```python
from build123d import *

# Parameters (mm, degrees)
F0_R     = 4.7879
F1_DEPTH = 15
F4_D     = 4.1
F5_D     = 4.1


with BuildPart() as f1:
    # F0 (on Top) → F1 (new body)
    with BuildSketch(Plane.XY):
        with BuildLine():
            ThreePointArc((-9.7879, 0), (0, 9.7879), (9.7879, 0))
            Line((9.7879, 0), (9.7879, 17.5))
            Line((9.7879, 17.5), (21.7879, 17.5))
            Line((21.7879, 17.5), (21.7879, 20))
            Line((21.7879, 20), (0, 20))
            Line((0, 20), (-21.7879, 20))
            Line((-21.7879, 20), (-21.7879, 17.5))
            Line((-21.7879, 17.5), (-9.7879, 17.5))
            Line((-9.7879, 17.5), (-9.7879, 0))
        make_face()
        with BuildLine():
            ThreePointArc((-9.7879, 0), (0, -9.7879), (9.7879, 0))
            ThreePointArc((9.7879, 0), (0, 9.7879), (-9.7879, 0))
        make_face()
        Circle(F0_R, mode=Mode.SUBTRACT)
    extrude(amount=F1_DEPTH)

    # F4 (through all)
    with Locations(Plane.XZ.offset(-17.5)):
        with Locations((15.7879, 7.5)):
            Hole(F4_D / 2)

    # F5 (through all)
    with Locations(Plane.XZ.offset(-17.5)):
        with Locations((-15.7879, 7.5)):
            Hole(F5_D / 2)


solid = f1.part
```
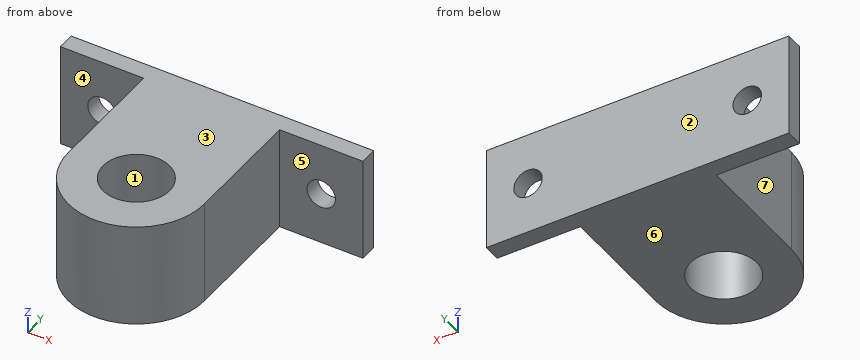
Design review of the part built by this model. Coordinates are the model's own, in mm. Face numbers are marked on the shaded views. A direction names the side the tool comes from. Coordinates: 2 decimals unless noted, no trailing zeros. Write each loop counter-clockwise with the first axis right and the second up, starting at its lowest first coordinate (ties: lowest second). Pieces come first, ordered by that corner, then holes.
1) Add section D-D (y = 2.5). Write out the cut boundary in (x, z).
2) Add section B-B (x = 0). Write out the cut boundary in (y, z).
3) Machinability: for the marked faces 5, 6 and 7, which of the approach directions +Z, -Z, +X, -X, +Y, -Y give a long, thin tool a straight path to every point of the face, cutting with its end or side? Answer none if there is none.
4) Add section C-C (z = 3). Write out the cut boundary in (x, y), plus the area to 3 significant figures.
5) To check wall thickness, follow L1, parallel to Y at x = 0, z = 4.25; L2, parallel to X at y = 2, z = 10.25; L3, parallel to Y at x = 19.5, z = 13. State the ranges of each line that lie inside material, in increasing order.
6) Mouldability with a two-part tool opening along Y and no side actions: class the marked faces 1, 2, 3 and 4 as +Y half, -Y half, draft (parallel to the pull), parting line (faces both ways), or undercut.
7) Add section A-A (z = 7.5). Write out the cut boundary in (x, y).
8) Insertion check: pin 1 (5 mm diameter, centred on x = 7, z = 8.5, fed in from -Y); pin 2 (4 mm diameter, centred on y = 17, z = 5.5, fed in from -X); pin 3 (6 mm diameter, centred on x = -17.5, z = 10.5, fed in from -Y); pin 4 (4 mm diameter, centred on y = 1.5, z = 2.5, fed in from -X). Each pin has a flat end and moves straight along its axis. Give the tip position at first contact, or say it passes through.
Check result:
1. outline: (-9.79, 0) - (-4.08, 0) - (-4.08, 15) - (-9.79, 15) - close; (4.08, 0) - (9.79, 0) - (9.79, 15) - (4.08, 15) - close
2. outline: (-9.79, 0) - (-4.79, 0) - (-4.79, 15) - (-9.79, 15) - close; (4.79, 0) - (20, 0) - (20, 15) - (4.79, 15) - close
3. face 5: +Z, -Z, +X, -Y
3. face 6: -Z, +X, -X, +Y, -Y
3. face 7: +Z, -Z, -X, -Y
4. outline: (-21.79, 17.5) - (-9.79, 17.5) - (-9.79, 0) arc R9.79 ccw to (9.79, 0) - (9.79, 17.5) - (21.79, 17.5) - (21.79, 20) - (-21.79, 20) - close; hole circle Ø9.58 at (0, 0)
4. area: 530 mm2
5. L1: y = -9.79 to -4.79, 4.79 to 20
5. L2: x = -9.79 to -4.35, 4.35 to 9.79
5. L3: y = 17.5 to 20
6. face 1: undercut
6. face 2: +Y half
6. face 3: draft
6. face 4: -Y half
7. outline: (-21.79, 17.5) - (-17.84, 17.5) - (-17.84, 20) - (-21.79, 20) - close; (-13.74, 17.5) - (-9.79, 17.5) - (-9.79, 0) arc R9.79 ccw to (9.79, 0) - (9.79, 17.5) - (13.74, 17.5) - (13.74, 20) - (-13.74, 20) - close; (17.84, 17.5) - (21.79, 17.5) - (21.79, 20) - (17.84, 20) - close; hole circle Ø9.58 at (0, 0)
8. pin 1: stops at y = -8.69
8. pin 2: stops at x = -21.79
8. pin 3: stops at y = 17.5
8. pin 4: stops at x = -9.79
